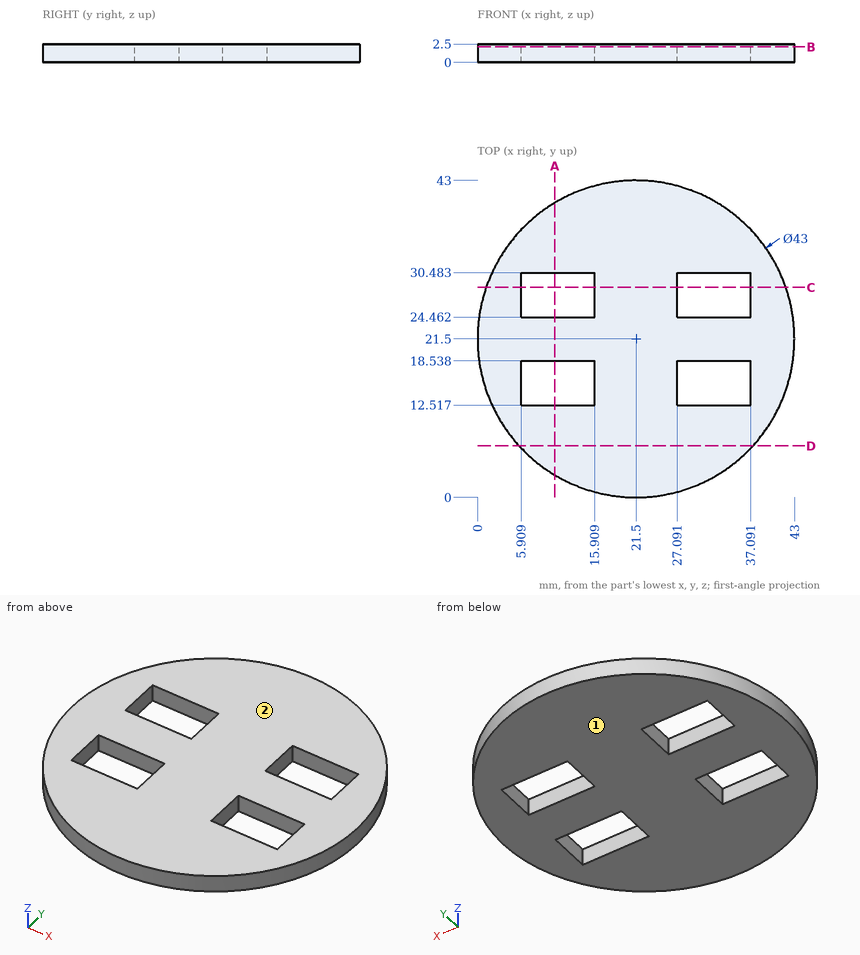
Can you work these out from the drawing? Everything is in mm from the part's minimum corner. Coordinates: 2 decimals unless noted, no trailing zeros. Loops run counter-clockwise (first coordinate to the right, second up) from the corner with the lowest first, then second, coordinate; pieces in that order, holes last.
1. For P1, Ø1.2, axis at x = 34, z = 1.5, coming from the +Y side; P2, Ø0.8, axis at x = 33, z = 1, coming from the +Y side; P3, Ø0.8, axis at x = 9.5, z = 1.5, coming from the +Y side, each with a flat end and sliding along its axis, tell me the tip position at first contact or that it passes through.
2. Imagine slicing it at A-A, the plane x = 10.5. Please give me the cut outline in (y, z).
3. Imagine slicing it at B-B, the plane z = 2.1. Please give me the cut outline in (x, y).
4. I need wall thicknesses on L1, parallel to Y at x = 15, z = 1.65 (1 decimal); L2, parallel to X at y = 28, z = 2.1 (1 decimal); L3, parallel to Y at x = 10.5, z = 1.3. Which ranges of each line are inside material? Lowest first, please.
5. If we mould it in two halves opening along Z, with no side actions, what happens to the marked faces 1 and 2? For each: pulls with the +Z half, pulls with the -Z half, needs draft (parallel to the pull), parting line crosses it, or undercut.
6. Imagine slicing it at C-C, the plane y = 28.5. Please give me the cut outline in (x, z).
7. Imagine slicing it at D-D, the plane y = 7. Please give me the cut outline in (x, z) (1 decimal).
Taken from the geometry:
1. P1: stops at y = 39.41
1. P2: stops at y = 39.91
1. P3: stops at y = 39.6
2. outline: (3.03, 0) - (12.52, 0) - (12.52, 2.5) - (3.03, 2.5) - close; (18.54, 0) - (24.46, 0) - (24.46, 2.5) - (18.54, 2.5) - close; (30.48, 0) - (39.97, 0) - (39.97, 2.5) - (30.48, 2.5) - close
3. outline: circle Ø43 at (21.5, 21.5); hole (5.91, 12.52) - (15.91, 12.52) - (15.91, 18.54) - (5.91, 18.54) - close; hole (5.91, 24.46) - (15.91, 24.46) - (15.91, 30.48) - (5.91, 30.48) - close; hole (27.09, 12.52) - (37.09, 12.52) - (37.09, 18.54) - (27.09, 18.54) - close; hole (27.09, 24.46) - (37.09, 24.46) - (37.09, 30.48) - (27.09, 30.48) - close
4. L1: y = 1 to 12.5, 18.5 to 24.5, 30.5 to 42
4. L2: x = 1 to 5.9, 15.9 to 27.1, 37.1 to 42
4. L3: y = 3.03 to 12.52, 18.54 to 24.46, 30.48 to 39.97
5. face 1: pulls with the -Z half
5. face 2: pulls with the +Z half
6. outline: (1.17, 0) - (5.91, 0) - (5.91, 2.5) - (1.17, 2.5) - close; (15.91, 0) - (27.09, 0) - (27.09, 2.5) - (15.91, 2.5) - close; (37.09, 0) - (41.83, 0) - (41.83, 2.5) - (37.09, 2.5) - close
7. outline: (5.6, 0) - (37.4, 0) - (37.4, 2.5) - (5.6, 2.5) - close
